from build123d import *

# Parameters (mm, degrees)
SKETCH5_W           = 50
SKETCH5_H           = 84.944653118
SKETCH5_W_2         = 40
SKETCH5_H_2         = 20
BOSS_EXTRUDE1_DEPTH = 5


with BuildPart() as part:
    # Sketch5 → Boss-Extrude1 (new body)
    with BuildSketch(Plane.XY):
        Polygon((-110, 120), (-120, 120), (-120, 110), (-125, 110), (-125, 80), (-120, 80), (-120, 15), (-125, 15), (-125, -15), (-120, -15), (-120, -80), (-125, -80), (-125, -110), (-120, -110), (-120, -120), (-110, -120), (-110, -125), (-80, -125), (-80, -120), (-15, -120), (-15, -125), (15, -125), (15, -120), (80, -120), (80, -125), (110, -125), (110, -120), (120, -120), (120, -110), (125, -110), (125, -80), (120, -80), (120, -15), (125, -15), (125, 15), (120, 15), (120, 80), (125, 80), (125, 110), (120, 110), (120, 120), (110, 120), (110, 125), (80, 125), (80, 120), (15, 120), (15, 125), (-15, 125), (-15, 120), (-80, 120), (-80, 125), (-110, 125), align=None)
        with Locations((-45, 0)):
            Rectangle(SKETCH5_W, SKETCH5_H, mode=Mode.SUBTRACT)
        with Locations((10, 0)):
            Rectangle(SKETCH5_W_2, SKETCH5_H_2, mode=Mode.SUBTRACT)
    extrude(amount=BOSS_EXTRUDE1_DEPTH)


solid = part.part
Here's how the part is built. I have some questions about the finished solid (model axes, mm). Coordinates: 2 decimals unless noted, no trailing zeros. Order: outer loops, then holes, each group sorted by start corner. A loop starts at its lowest first (then second) coordinate and runs counter-clockwise, first axis right, second up. Notation, with made-up numbers: (86.5, -30.75) - (128.5, -30.75) arc R7 ccw to (128.5, -24.75) - close; hole circle Ø11 at (18.5, 17). An arc over 180 degrees is marked (long way). Use CSV: the item, a comma, the result in double quotes. Start each with the question number.
1. Suppose I cut it at A-A on y = 20. List the corners of the cut face in (x, z) for me, then the cut area to 3 significant figures.
2. I'm going to push flat-ended pins straight in: pin 1 (2.5 mm diameter, centred on x = 123, z = 3.5, fed in from +Y); pin 2 (2.5 mm diameter, centred on x = 114, z = 2.5, fed in from -Y); pin 3 (1.5 mm diameter, centred on y = -122, z = 3.5, fed in from +X). Where does each tip first touch, or does it pass through?
3. Suppose I cut it at B-B on x = -41. List the corners of the cut face in (y, z) for me, then the cut area to 3 significant figures.
4. Please list where these lines run through material, in increasing order: line 1 (X direction, y = 37, z = 1.55); line 2 (X direction, y = -9.5, z = 1.25); line 3 (Y direction, x = -47, z = 1.75). Write a range as from..to.
5. Suppose I cut it at C-C on x = 45.5. List the corners of the cut face in (y, z) for me.
6. Suppose I cut it at D-D on z = 2.5. Give the number of separate pieces and of enclosed holes in the cut face, then the cut area to 3 significant figures.
Output:
1,outline,"(-120, 0) - (-70, 0) - (-70, 5) - (-120, 5) - close; (-20, 0) - (120, 0) - (120, 5) - (-20, 5) - close"
1,area,"950 mm2"
2,pin 1,"stops at y = 110"
2,pin 2,"stops at y = -120"
2,pin 3,"stops at x = 110"
3,outline,"(-120, 0) - (-42.47, 0) - (-42.47, 5) - (-120, 5) - close; (42.47, 0) - (120, 0) - (120, 5) - (42.47, 5) - close"
3,area,"775 mm2"
4,line 1,"x = -120..-70, -20..120"
4,line 2,"x = -125..-70, -20..-10, 30..125"
4,line 3,"y = -120..-42.47, 42.47..120"
5,outline,"(-120, 0) - (120, 0) - (120, 5) - (-120, 5) - close"
6,separate pieces,"1"
6,enclosed holes,"2"
6,area,"54,400 mm2"
